Could you check a few things on this model? Use its own coordinates, in mm. A direction names the side the tool comes from. Round coordinates to 2 decimals unless told otherwise and drop trailing zeros. Loops run counter-clockwise (first coordinate to the right, second up) from the corner with the lowest first, then second, coordinate; pieces in that order, holes last. Notation, with made-up numbers: (62.5, 23.5) -> (113.5, 23.5) arc R20 cw to (113.5, 52.5) -> close; hole circle Ø10 at (22, 85). An arc over 180 degrees is marked (long way). One line per item, written item: value.
```python
from build123d import *

# Parameters (mm, degrees)
MODEL_R         = 1
EXTRUDE_1_DEPTH = 2


with BuildPart() as part:
    # Model → Бобышка-Вытянуть1 (new body)
    with BuildSketch(Plane.XY):
        with BuildLine():
            Line((15, 20), (24, 20))
            Line((24, 20), (24, 23))
            Line((24, 23), (34, 23))
            Line((34, 23), (34, -13))
            Line((34, -13), (24, -13))
            Line((24, -13), (24, -10))
            Line((24, -10), (15, -10))
            Line((15, -10), (15, -6))
            ThreePointArc((15, -6), (13.242640687, -1.757359313), (9, 0))
            Line((9, 0), (-9, 0))
            ThreePointArc((-9, 0), (-13.242640687, -1.757359313), (-15, -6))
            Line((-15, -6), (-15, -10))
            Line((-15, -10), (-24, -10))
            Line((-24, -10), (-24, -13))
            Line((-24, -13), (-34, -13))
            Line((-34, -13), (-34, 23))
            Line((-34, 23), (-24, 23))
            Line((-24, 23), (-24, 20))
            Line((-24, 20), (-15, 20))
            Line((-15, 20), (-15, 16))
            ThreePointArc((-15, 16), (-13.242640687, 11.757359313), (-9, 10))
            Line((-9, 10), (9, 10))
            ThreePointArc((9, 10), (13.242640687, 11.757359313), (15, 16))
            Line((15, 16), (15, 20))
        make_face()
        with Locations((30, -4)):
            Circle(MODEL_R, mode=Mode.SUBTRACT)
        with Locations((30, 14)):
            Circle(MODEL_R, mode=Mode.SUBTRACT)
        with Locations((-30, 14)):
            Circle(MODEL_R, mode=Mode.SUBTRACT)
        with Locations((-30, -4)):
            Circle(MODEL_R, mode=Mode.SUBTRACT)
    extrude(amount=EXTRUDE_1_DEPTH)


solid = part.part
```
(1) Imagine slicing it at D-D on y = 14. Write out the boundary of the cut face in (x, z).
Results below:
outline: (-34, 0) -> (-31, 0) -> (-31, 2) -> (-34, 2) -> close; (-29, 0) -> (-14.66, 0) -> (-14.66, 2) -> (-29, 2) -> close; (14.66, 0) -> (29, 0) -> (29, 2) -> (14.66, 2) -> close; (31, 0) -> (34, 0) -> (34, 2) -> (31, 2) -> close
(2) Imagine slicing it at B-B on x = 30. Write out the boundary of the cut face in (y, z), then the cut area to 3 significant figures.
Results below:
outline: (-13, 0) -> (-5, 0) -> (-5, 2) -> (-13, 2) -> close; (-3, 0) -> (13, 0) -> (13, 2) -> (-3, 2) -> close; (15, 0) -> (23, 0) -> (23, 2) -> (15, 2) -> close
area: 64.0 mm²
(3) Imagine slicing it at A-A on y = 19. Write out the boundary of the cut face in (x, z).
Results below:
outline: (-34, 0) -> (-15, 0) -> (-15, 2) -> (-34, 2) -> close; (15, 0) -> (34, 0) -> (34, 2) -> (15, 2) -> close
(4) For pin 1 Ø1 at (x, z) = (18, 0.5) entering from -Y, with a flat end and sliding along its axis, tell me the tip position at first contact or that it passes through.
Results below:
pin 1: stops at y = -10
(5) On a 3-axis mill with a long thin cutter (end or side, diameter ignored), from which of +Z, -Z, +X, -X, +Y, -Y can I reach the whole of each face in a straight line? I mean faces 5 (the face through (-13.289, 11.804, 0.986)), 6 (the face through (30, 13, 1)), 7 (the face through (-19, -10, 1)). Say none if no direction works.
Results below:
face 5: +Z, -Z, +Y
face 6: +Z, -Z
face 7: +Z, -Z, -Y
(6) We'd pull the mould along X, two halves only. Please class faces 1 (the face through (-34, 5, 1)), 2 (the face through (34, 5, 1)), 3 (the face through (-15, 18, 1)), 4 (the face through (15, 18, 1)): +X half, -X half, draft (parallel to the pull), parting line (faces both ways), or undercut.
Results below:
face 1: -X half
face 2: +X half
face 3: undercut
face 4: undercut
(7) Imagine slicing it at C-C on z = 1.1. Write out the boundary of the cut face in (x, y), then the cut area to 3 significant figures.
Results below:
outline: (-34, -13) -> (-24, -13) -> (-24, -10) -> (-15, -10) -> (-15, -6) arc R6 cw to (-9, 0) -> (9, 0) arc R6 cw to (15, -6) -> (15, -10) -> (24, -10) -> (24, -13) -> (34, -13) -> (34, 23) -> (24, 23) -> (24, 20) -> (15, 20) -> (15, 16) arc R6 cw to (9, 10) -> (-9, 10) arc R6 cw to (-15, 16) -> (-15, 20) -> (-24, 20) -> (-24, 23) -> (-34, 23) -> close; hole circle Ø2 at (-30, -4); hole circle Ø2 at (-30, 14); hole circle Ø2 at (30, -4); hole circle Ø2 at (30, 14)
area: 1,580 mm²
(8) Please list where these lines run through material, in increasing order: L1, parallel to Y at x = -30, z = 0.4; L2, parallel to X at y = -7.5, z = 1.9; L3, parallel to X at y = 20.5, z = 1.65.
Results below:
L1: y = -13 to -5, -3 to 13, 15 to 23
L2: x = -34 to -15, 15 to 34
L3: x = -34 to -24, 24 to 34
